Could you check a few things on this model? Use its own coordinates, in mm. Coordinates: 2 decimals unless noted, no trailing zeros. Loops run counter-clockwise (first coordinate to the right, second up) from the corner with the lowest first, then second, coordinate; pieces in that order, holes last. Notation, with made-up numbers: (89.25, -11) -> (114.25, -11) arc R30 cw to (114.25, 28) -> close; hole circle Ø11 at (9, -20). An arc over 180 degrees is marked (long way). One line per question, with ' | ' between items. Start each with the question number.
(1) Suppose I cut it at C-C (y = 3.5). Please give me the cut outline in (x, z), plus the area to 3 significant figures.
(2) Suppose I cut it at A-A (x = -4). Please give me the cut outline in (y, z).
(3) Suppose I cut it at B-B (z = 70). Please give me the cut outline in (x, y), plus the area to 3 significant figures.
(4) If we mould it in two halves opening along X, with no side actions, what happens to faces 1 (the face through (-4, 0, 65)), 2 (the face through (-8, 4, 65)), 3 (the face through (-4.09, 3.94, 67.9))? For each: pulls with the +X half, pulls with the -X half, needs draft (parallel to the pull), parting line crosses it, or undercut.
(5) If I drill on line 1 along Z through (x, y) = (-4, 3); line 2 along X through (y, z) = (4.5, 70); line 3 along Z through (x, y) = (-3, 3.75), over which ranges is the centre line in solid material (lowest first)?
Autodesk Inventor part; units mm, degrees
ref_plane "Plano de trabajo2" through (-29.9, -56.9, 56) normal (0, 0, -1) x (0, 1, 0)
ref_plane "YZ Plane" through (0, 0, 0) normal (1, 0, 0) x (0, 1, 0)
ref_plane "XZ Plane" through (0, 0, 0) normal (0, 1, 0) x (-1, 0, 0)
sketch "Boceto1" plane through (0, 0, 0) normal (0, 1, 0) x (-1, 0, 0)
  line L0 (0, 0) -> (8, 0)
  line L1 (8, 0) -> (8, 66)
  line L2 (8, 66) -> (0, 66)
  line L3 (0, 66) -> (0, 0)
  dimension "d0" = 8
  dimension "d1" = 66
extrude "Extrusión1" add sketch "Boceto1" along normal blind 8
ref_plane "Plano de trabajo1" through (-12.4, -21.9, 10) normal (0, 0, 1) x (1, 0, 0)
sketch "Boceto2" plane through (-12.4, -21.9, 10) normal (0, 0, 1) x (1, 0, 0)
  line L0 (4.4, 21.9) -> (12.4, 21.9)
  line L1 (12.4, 21.9) -> (12.4, 29.9)
  line L2 (4.4, 29.9) -> (12.4, 29.9)
  line L3 (4.4, 21.9) -> (4.4, 29.9)
  line L4 (3.4, 30.9) -> (13.4, 30.9)
  line L5 (13.4, 30.9) -> (13.4, 20.9)
  line L6 (13.4, 20.9) -> (3.4, 20.9)
  line L7 (3.4, 20.9) -> (3.4, 30.9)
  line L8 (4.4, 21.9) -> (3.4, 21.9)
  line L9 (12.4, 21.9) -> (13.4, 21.9)
  dimension "d23" = 1
ref_plane "Plano de trabajo2" through (-29.9, -56.9, 56) normal (0, 0, -1) x (0, 1, 0)
extrude "Extrusión2" add sketch "Boceto2" along normal up to surface (46 mm away) contours L8 L7 L4 L5 L9 L1 L2 L3
sketch "Boceto3" plane through (-8, 0, 66) normal (0, 0, 1) x (1, 0, 0)
  line L0 (0, 0) -> (8, 0)
  line L1 (8, 0) -> (8, 8)
  line L2 (0, 8) -> (8, 8)
  line L3 (0, 0) -> (0, 8)
extrude "Extrusión3" add sketch "Boceto3" along normal blind 8
sketch "Boceto4" plane through (0, 0, 0) normal (0, 0, -1) x (-1, 0, 0)
  line L0 (0, 0) -> (8, 0)
  line L1 (8, 0) -> (8, 8)
  line L2 (0, 8) -> (8, 8)
  line L3 (0, 0) -> (0, 8)
extrude "Extrusión4" add sketch "Boceto4" along normal blind 8
sketch "Boceto5" plane through (0, 8, 0) normal (0, 1, 0) x (1, 0, 0)
  line L0 (-8, -10) -> (-8, 8)
  line L1 (0, -74) -> (-8, -74)
  line L2 (0, -56) -> (0, -74)
  line L3 (-8, 8) -> (0, 8)
  line L4 (0, 8) -> (-8, 8)
  line L5 (-8, 8) -> (-8, 0)
  line L6 (-8, 0) -> (0, 0)
  line L7 (0, 0) -> (0, 8)
  line L8 (0, -74) -> (-8, -74)
  line L9 (-8, -74) -> (-8, -66)
  line L10 (-8, -66) -> (0, -66)
  line L11 (0, -66) -> (0, -74)
  line L12 (0, 8) -> (-8, 0)
  line L13 (0, -74) -> (-8, -66)
  circle A0 centre (-4, 4) radius 2.1
  circle A1 centre (-4, -70) radius 2.1
  line L14 (-8, -10) -> (0, -10)
  line L15 (0, -10) -> (0, 8)
  line L16 (0, -56) -> (-8, -56)
  line L17 (-8, -56) -> (-8, -74)
  point P0 (0, 0)
  dimension "d11" = 4.2
  dimension "d12" = 4.2
  dimension "d13" = 8
  dimension "d14" = 8
hole "Agujero1" at (-4, 8, -4) at (-4, 8, 70) direction (0, -1, 0) diameter 4.2 end through all
ref_plane "Plano de trabajo3" through (-12.4, -15.4, 56) normal (0, 0, -1) x (-1, 0, 0)
split "Dividir1" plane through (-12.4, -15.4, 56) removes the side toward (0, 0, -1)
properties part number "Refuerzo superior"
Checks:
1) outline: (-8, 56) -> (0, 56) -> (0, 74) -> (-8, 74) -> close; hole circle Ø4.2 at (-4, 70) | area: 130 mm^2
2) outline: (0, 56) -> (8, 56) -> (8, 67.9) -> (0, 67.9) -> close; (0, 72.1) -> (8, 72.1) -> (8, 74) -> (0, 74) -> close
3) outline: (-8, 0) -> (-6.1, 0) -> (-6.1, 8) -> (-8, 8) -> close; (-1.9, 0) -> (0, 0) -> (0, 8) -> (-1.9, 8) -> close | area: 30.4 mm^2
4) face 1: needs draft | face 2: pulls with the -X half | face 3: undercut
5) line 1: z = 56 to 67.9, 72.1 to 74 | line 2: x = -8 to -6.1, -1.9 to 0 | line 3: z = 56 to 68.15, 71.85 to 74
